Here's how the part is built. I have some questions about the finished solid (model axes, mm). A direction names the side the tool comes from. Give positions to 0.01 mm unless a question says otherwise; leave off trailing zeros. Write each loop counter-clockwise with the first axis right and the second up, starting at its lowest first coordinate (ties: lowest second). Pieces come first, ordered by that corner, then holes. Notation, with made-up numbers: (36.5, 76.25) - (83.5, 76.25) arc R22 ccw to (83.5, 110.25) - close; hole circle Ø8 at (57.25, -28.75). An arc over 180 degrees is marked (long way). Write each question's results on one line, items separated by ' | '. Start each with the question number.
Item 1: Which directions (+Z, -Z, +X, -X, +Y, -Y) give clear straight access to the entire face, cutting with the end or side of a thin tool? Please do faces 4 (the cylindrical face through (31.243, 1.006, -19.716)), 5 (the flat face through (-32, 1.984, -13)).
Item 2: Please list where these lines run through material, in increasing order: line 1 along X through (y, z) = (1, -19); line 2 along X through (y, z) = (0.55, -19.25); line 3 along X through (y, z) = (25, -0.5).
Item 3: We'd pull the mould along X, two halves only. Please class faces 1 (the cylindrical face through (0.65, 1.01, -36.45)), 2 (the flat face through (25.4, 0, -19.4)), 3 (the cylindrical face through (42.174, 1.006, 9.365)): +X half, -X half, draft (parallel to the pull), parting line (faces both ways), or undercut.
Item 4: Suppose I cut it at D-D on x = -23. List the corners of the cut face in (y, z) for me (1 decimal), then the cut area to 3 significant figures.
Item 5: Will these pins go through, and if not, where does the flat tip stop? P1, Ø10, axis at y = 16, z = -19, coming from the +X side; P2, Ø1.5, axis at x = 13.5, z = 19, coming from the -Y side; P3, Ø2, axis at x = 21.5, y = 22, coming from the -Z side.
Item 6: Suppose I cut it at B-B on z = 38.5. List the corners of the cut face in (x, y) for me, then the cut area to 3 significant figures.
```python
from build123d import *

# Parameters (mm, degrees)
SKETCH2_R          = 2.15
CUT_EXTRUDE1_DEPTH = 10


with BuildPart() as part:
    # Sketch1 → Revolve1 (revolve)
    with BuildSketch(Plane(origin=(0, 0, 0), x_dir=(0, 0, -1), z_dir=(1, 0, 0)), mode=Mode.PRIVATE) as revolve1_sk:
        with BuildLine():
            Line((-31.75, 0), (-43.200960454, 0))
            Line((-43.200960454, 0), (-43.200960454, 1.984375))
            Line((-43.200960454, 1.984375), (-33.675960454, 1.984375))
            ThreePointArc((-33.675960454, 1.984375), (-23.141590333, 24.545363178), (0, 33.734375))
            Line((0, 33.734375), (0, 31.75))
            ThreePointArc((0, 31.75), (-22.450640303, 22.450640303), (-31.75, 0))
        make_face()
    revolve(revolve1_sk.sketch.rotate(Axis((0, -1000, 0), (0, 1, 0)), 180), axis=Axis((0, -1000, 0), (0, 1, 0)))

    # Sketch2 → Cut-Extrude1 (cut)
    with BuildSketch(Plane(origin=(0, 1.984375, 0), x_dir=(1, 0, 0), z_dir=(0, 1, 0))):
        with Locations(Location((0, -38.5, 0), (0, 0, 270))):
            Circle(SKETCH2_R)
        with Locations(Location((-33.341978046, -19.25, 0), (0, 0, 270))):
            Circle(SKETCH2_R)
        with Locations(Location((-33.341978046, 19.25, 0), (0, 0, 270))):
            Circle(SKETCH2_R)
        with Locations(Location((0, 38.5, 0), (0, 0, 270))):
            Circle(SKETCH2_R)
        with Locations(Location((33.341978046, 19.25, 0), (0, 0, 270))):
            Circle(SKETCH2_R)
        with Locations(Location((33.341978046, -19.25, 0), (0, 0, 270))):
            Circle(SKETCH2_R)
    extrude(amount=-CUT_EXTRUDE1_DEPTH, mode=Mode.SUBTRACT)


solid = part.part
```
Checked values:
1) face 4: +Y, -Y | face 5: +Y
2) line 1: x = -38.8 to -35.48, -31.21 to -25.42, 25.42 to 31.21, 35.48 to 38.8 | line 2: x = -38.68 to -35.49, -31.19 to -25.24, 25.24 to 31.19, 35.49 to 38.68 | line 3: x = -22.64 to -19.57, 19.57 to 22.64
3) face 1: undercut | face 2: draft | face 3: parting line
4) outline: (0, -36.6) - (2, -36.6) - (2, -24.6) arc R24.7 ccw to (2, 24.6) - (2, 36.6) - (0, 36.6) - (0, 21.9) arc R21.9 cw to (0, -21.9) - close | area: 251 mm^2
5) P1: stops at x = 27.28 | P2: stops at y = 20.72 | P3: stops at z = -15.88
6) outline: (-19.6, 0) - (-2.15, 0) - (-2.15, 1.98) - (-19.6, 1.98) - close; (2.15, 0) - (19.6, 0) - (19.6, 1.98) - (2.15, 1.98) - close | area: 69.2 mm^2
